Can you work these out from the model? Positions are in its coordinate system, mm. Face numbers are marked on the shaded views. A direction names the side the tool comes from. Round coordinates to 2 decimals unless told otherwise and drop trailing zeros. Order: outer loops, then holes, each group sorted by start corner. A loop starts at its lowest first (then second) coordinate and runs counter-clockwise, first axis right, second up. Notation, with made-up numbers: M 39,58.5 L 65,58.5 A17 ccw 65,63.5 Z; hole C 1.5,68 d7. An arc over 180 degrees is marked long. Answer as CSV lines item,"result". Start each with the question number.
from build123d import *

# Parameters (mm, degrees)
SM_BASE_FLANGE_1_DEPTH = 2
SKETCH_8_R             = 1.6
CUT_EXTRUDE_1_DEPTH    = 10
FILLET_1_R             = 3
OTHER_START            = 6.58904
OTHER_1_OUTLINE_W      = 8
OTHER_1_OUTLINE_H      = 2
OTHER_1_DEPTH          = 15.41096
OTHER_START_2          = 5
OTHER_1_2_OUTLINE_R    = 1.6
OTHER_1_2_DEPTH        = 0.473479212
OTHER_START_3          = 6.529597681
OTHER_1_3_OUTLINE_W    = 8
OTHER_1_3_OUTLINE_H    = 2
OTHER_1_3_DEPTH        = 0.059442319
OTHER_START_4          = 3
OTHER_1_4_OUTLINE_R    = 1.6
OTHER_1_4_DEPTH        = 4
OTHER_1_5_OUTLINE_W    = 23
OTHER_1_5_OUTLINE_H    = 2
OTHER_1_5_DEPTH        = 0.46188997
OTHER_START_5          = -15.5
OTHER_1_6_DEPTH        = 31
OTHER_START_6          = -7.5
OTHER_1_7_DEPTH        = 23
OTHER_1_8_DEPTH        = 23


with BuildPart() as part:
    # 基体-法兰1: sheet metal written as solids
    # Sketch 1 → 基体-法兰1 (new body)
    with BuildSketch(Plane(origin=(0, 0, 0), x_dir=(1, 0, 0), z_dir=(0, 1, 0))):
        Polygon((-7.5, -5), (15.5, -5), (15.5, 5), (-15.5, 5), (-15.5, -5), (-15.5, -22), (-7.5, -22), align=None)
    extrude(amount=-SM_BASE_FLANGE_1_DEPTH)

    # 草图8 → 切除-拉伸1 (cut)
    with BuildSketch(Plane.XZ.offset(2)):
        with Locations(Location((-11.5, 18.5, 0), (0, 0, 270))):
            Circle(SKETCH_8_R)
        with Locations(Location((-11.5, 10.5, 0), (0, 0, 270))):
            Circle(SKETCH_8_R)
    extrude(amount=-CUT_EXTRUDE_1_DEPTH, mode=Mode.SUBTRACT)

    # 圆角1
    fillet_1_edges = [part.edges().sort_by_distance(p)[0] for p in [
        (15.5, -1, -5),
        (-15.5, -1, -5),
        (-15.5, -1, 22),
        (-7.5, -1, 22),
    ]]
    fillet(fillet_1_edges, radius=FILLET_1_R)

    # Other 1: read off the stored shape, not the designer's step
    # Other 1 outline → Other 1 (cut)
    with BuildSketch(Plane.XY.offset(OTHER_START)):
        with Locations((-11.5, -1)):
            Rectangle(OTHER_1_OUTLINE_W, OTHER_1_OUTLINE_H)
    extrude(amount=OTHER_1_DEPTH, mode=Mode.SUBTRACT)

    # Other 1 2 outline → Other 1 2 (add)
    with BuildSketch(Plane.XY.offset(OTHER_START_2)):
        with BuildLine():
            Line((-7.5, -15.28761102), (-7.5, -2))
            Line((-7.5, -2), (-15.5, -2))
            Line((-15.5, -2), (-15.5, -15.28761102))
            ThreePointArc((-15.5, -15.28761102), (-14.621320344, -17.408931363), (-12.5, -18.28761102))
            Line((-12.5, -18.28761102), (-10.5, -18.28761102))
            ThreePointArc((-10.5, -18.28761102), (-8.378679656, -17.408931364), (-7.5, -15.28761102))
        make_face()
        with Locations((-11.5, -14.78761102)):
            Circle(OTHER_1_2_OUTLINE_R, mode=Mode.SUBTRACT)
        with Locations((-11.5, -6.78761102)):
            Circle(OTHER_1_2_OUTLINE_R, mode=Mode.SUBTRACT)
    extrude(amount=OTHER_1_2_DEPTH)

    # Other 1 3 outline → Other 1 3 (cut)
    with BuildSketch(Plane.XY.offset(OTHER_START_3)):
        with Locations((-11.5, -1)):
            Rectangle(OTHER_1_3_OUTLINE_W, OTHER_1_3_OUTLINE_H)
    extrude(amount=OTHER_1_3_DEPTH, mode=Mode.SUBTRACT)

    # Other 1 4 outline → Other 1 4 (add)
    with BuildSketch(Plane.XY.offset(OTHER_START_4)):
        with BuildLine():
            Line((-7.5, -15.28761102), (-7.5, -2))
            Line((-7.5, -2), (-15.5, -2))
            Line((-15.5, -2), (-15.5, -15.28761102))
            ThreePointArc((-15.5, -15.28761102), (-14.621320344, -17.408931363), (-12.5, -18.28761102))
            Line((-12.5, -18.28761102), (-10.5, -18.28761102))
            ThreePointArc((-10.5, -18.28761102), (-8.378679656, -17.408931364), (-7.5, -15.28761102))
        make_face()
        with Locations((-11.5, -14.78761102)):
            Circle(OTHER_1_4_OUTLINE_R, mode=Mode.SUBTRACT)
        with Locations((-11.5, -6.78761102)):
            Circle(OTHER_1_4_OUTLINE_R, mode=Mode.SUBTRACT)
    extrude(amount=OTHER_1_4_DEPTH)

    # Other 1 5 outline → Other 1 5 (add)
    with BuildSketch(Plane.XY.offset(OTHER_START_2)):
        with Locations((4, -1)):
            Rectangle(OTHER_1_5_OUTLINE_W, OTHER_1_5_OUTLINE_H)
    extrude(amount=OTHER_1_5_DEPTH)

    # Other 1 6 outline → Other 1 6 (cut)
    with BuildSketch(Plane.YZ.offset(OTHER_START_5)):
        with BuildLine():
            ThreePointArc((-2, 3), (-2.585786438, 4.414213562), (-4, 5))
            Line((-4, 5), (-18.28761102, 5))
            Line((-18.28761102, 5), (-18.28761102, 3))
            Line((-18.28761102, 3), (-2, 3))
        make_face()
        with BuildLine():
            Line((-2, 7), (-4, 7))
            ThreePointArc((-4, 7), (-1.171572875, 5.828427125), (0, 3))
            Line((0, 3), (0, 6.529597681))
            Line((0, 6.529597681), (-2, 6.529597681))
            Line((-2, 6.529597681), (-2, 7))
        make_face()
    extrude(amount=OTHER_1_6_DEPTH, mode=Mode.SUBTRACT)

    # Other 1 7 outline → Other 1 7 (cut)
    with BuildSketch(Plane.YZ.offset(OTHER_START_6)):
        Polygon((-2, 5.46188997), (-2, 4.573685779), (-0.871179745, 5.46188997), align=None)
    extrude(amount=OTHER_1_7_DEPTH, mode=Mode.SUBTRACT)

    # Other 1 8 outline → Other 1 8 (add)
    with BuildSketch(Plane.YZ.offset(OTHER_START_6)):
        with BuildLine():
            Line((-2, 4.573685779), (-2.428225479, 4.236739606))
            ThreePointArc((-2.428225479, 4.236739606), (-2.110086108, 3.654389393), (-2, 3))
            Line((-2, 3), (-2, 4.573685779))
        make_face()
        with BuildLine():
            Line((-0.856450957, 5.473479212), (-0.871179745, 5.46188997))
            Line((-0.871179745, 5.46188997), (-0.847366533, 5.46188997))
            ThreePointArc((-0.847366533, 5.46188997), (-0.851903412, 5.467688772), (-0.856450957, 5.473479212))
        make_face()
    extrude(amount=OTHER_1_8_DEPTH)


solid = part.part
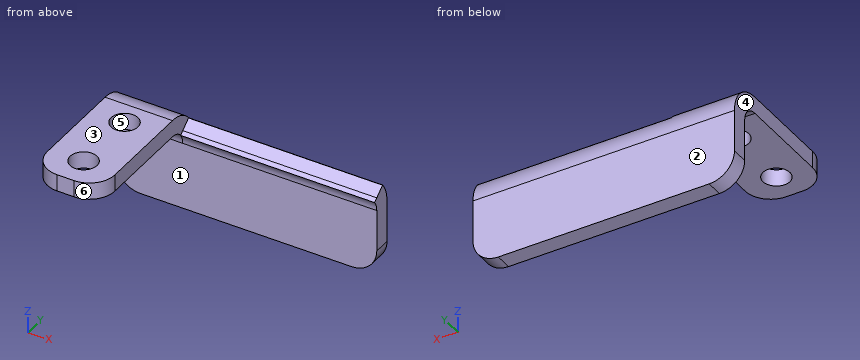
(1) If I drill on line 1 along Y through (x, z) = (-10.5, 5.5); line 2 along Y through (x, z) = (-11.5, 6.35); line 3 along Z through (x, y) = (-13, -12.5), over which ranges is the centre line in solid material (lowest first)?
(2) I want a section at A-A on x = -11.5. Write out the boundary of the cut face in (y, z), and give its area (3 significant figures).
(3) If we mould it in two halves opening along X, with no side actions, what happens to the marked faces 3, 4, 5 and 6? For each: +X half, -X half, draft (parallel to the pull), parting line (faces both ways), or undercut.
(4) I want a section at B-B on y = -9.5. Write out the boundary of the cut face in (x, z), and give its area (3 significant figures).
(5) I'm going to push flat-ended pins straight in: P1, Ø1.5, axis at x = 4.5, z = 2.5, coming from the -Y side; P2, Ø4, axis at x = -12, y = -14.5, coming from the -Z side; P3, Ø2, axis at y = -4.5, z = 6, coming from the +X side. Where does each tip first touch, or does it pass through?
(6) For the marked faces 1 and 2, which set-ups out of +Z, -Z, +X, -X, +Y, -Y let a thin tool reach every point of the face, with its end or its side?
(7) I want a section at D-D on z = 2. Write out the boundary of the cut face in (x, y), and give its area (3 significant figures).
From the geometry:
1,line 1,"-18.29 to -16.04, -13.54 to -8.04, -5.54 to -0.88"
1,line 2,"-18.29 to -16.39, -13.19 to -8.39, -5.19 to -1.81"
1,line 3,"5 to 7"
2,outline,"M -18.29,5 L -16.39,5 L -16.39,7 L -18.29,7 Z; M -13.19,5 L -8.39,5 L -8.39,7 L -13.19,7 Z; M -5.19,5 L -4,5 A2 cw -2,3 L -2,-5 L 0,-5 L 0,3 A4 ccw -4,7 L -5.19,7 Z"
2,area,"41.2 mm²"
3,face 3,"draft"
3,face 4,"-X half"
3,face 5,"undercut"
3,face 6,"+X half"
4,outline,"M -15.5,5 L -7.5,5 L -7.5,7 L -15.5,7 Z"
4,area,"16.0 mm²"
5,P1,"y = -2.02"
5,P2,"z = 5"
5,P3,"x = -7.5"
6,face 1,"-Z, +X, -X, -Y"
6,face 2,"+Z, -Z, +X, -X, +Y"
7,outline,"M -15.5,-2 L 15.5,-2 L 15.5,0 L -15.5,0 Z"
7,area,"62.0 mm²"
